Source: CAD feature listing. Evaluate the final solid. Frame: model axes, mm. A direction names the side the tool comes from. Give positions to 0.01 mm unless a question says otherwise; leave off trailing zeros. Loops run counter-clockwise (first coordinate to the right, second up) from the corner with the lowest first, then second, coordinate; pieces in that order, holes last. Notation, with made-up numbers: (-9.75, 9) -> (-2.75, 9) arc R26 cw to (-2.75, 44) -> close; hole circle Ø10 at (-26.75, 42.5). An arc over 180 degrees is marked (long way). Return JSON: item names as keys, results as strings. Group by question number.
(1) Cut plane A-A on x = -16.5. Return loops of the section in (y, z), then the cut area to 3 significant figures.
(2) Cut plane C-C on x = 0. Give the number of separate pieces and of enclosed holes in the cut face, then the cut area to 3 significant figures.
(3) Access query for faces 1 (the face through (52, 57, 10)), 2 (the face through (55, 10, 55)), 3 (the face through (-28, 57, 108)), 4 (the face through (23.944, 68.526, 104.028)). Directions: +Z, -Z, +X, -X, +Y, -Y. A direction counts if a zero-diameter tool reaches every point of the face in a straight line with its end or side. Return the directions, or none.
(4) Cut plane B-B on z = 52.5. Return loops of the section in (x, y), then the cut area to 3 significant figures.
(5) Cut plane D-D on y = -29.5. Return loops of the section in (x, z), then the cut area to 3 significant figures.
(6) Draft query along Y for faces 5 (the face through (-56.52, -9.85, 9.39)), 6 (the face through (-28, 57, 10)), 7 (the face through (-24.06, 67.65, 17)). Return one class per face: released by +Y, released by -Y, zero draft, split by the parting line, or undercut.
(7) Ray query, line 1 (X direction, y = 20.5, z = 59.5); line 2 (X direction, y = 65, z = 110); line 3 (Z direction, x = 20.5, y = 43.5). Return the intervals inside material, ascending. Write a range as from..to.
(8) Pin query (flat end, axial travel): pin 1 (6.5 mm diameter, centred on y = 58, z = 102, fed in from +X); pin 2 (7 mm diameter, centred on x = -4, y = -2, fed in from -Z); pin 3 (6 mm diameter, centred on y = 60.5, z = 110, fed in from -X). Return the tip coordinate at first contact, or that it passes through.
```python
from build123d import *

# Parameters (mm, degrees)
SKETCH_W        = 110
SKETCH_H        = 85
SKETCH_R        = 2.6
PAD_DEPTH       = 6
SKETCH001_R     = 12
POCKET_DEPTH    = 2
SKETCH002_W     = 110
SKETCH002_H     = 120
SKETCH002_W_2   = 75
SKETCH002_H_2   = 65
PAD001_DEPTH    = 6
PAD002_DEPTH    = 3
SKETCH004_W     = 8
SKETCH004_H     = 20
PAD003_DEPTH    = 22
SKETCH005_R     = 2.6
POCKET001_DEPTH = 110.001
FILLET_R        = 9.99
CHAMFER_SIZE    = 9.99
FILLET001_R     = 6
FILLET002_R     = 3
CHAMFER001_SIZE = 1.99
FILLET003_R     = 24


with BuildPart() as part:
    # Sketch → Pad (new body)
    with BuildSketch(Plane.XY):
        Rectangle(SKETCH_W, SKETCH_H)
        with Locations((0, -7.5)):
            Circle(SKETCH_R, mode=Mode.SUBTRACT)
    extrude(amount=PAD_DEPTH)

    # Sketch001 (on Face6 of Pad) → Pocket (cut)
    with BuildSketch(Plane(origin=(0, 0, 0), x_dir=(1, 0, 0), z_dir=(0, 0, -1))):
        with Locations((0, 7.5)):
            Circle(SKETCH001_R)
    extrude(amount=-POCKET_DEPTH, mode=Mode.SUBTRACT)

    # Sketch002 (on Face1 of Pocket) → Pad001 (join)
    with BuildSketch(Plane(origin=(0, 42.5, 0), x_dir=(-1, 0, 0), z_dir=(0, 1, 0))):
        with Locations((0, 60)):
            Rectangle(SKETCH002_W, SKETCH002_H)
        with Locations((0, 57.5)):
            Rectangle(SKETCH002_W_2, SKETCH002_H_2, mode=Mode.SUBTRACT)
    extrude(amount=PAD001_DEPTH)

    # Sketch003 (on Face15 of Pad001) → Pad002 (join)
    with BuildSketch(Plane.YZ.offset(55)):
        Polygon((-42.5, 6), (42.5, 120), (48.5, 120), (48.5, 0), (-42.5, 0), align=None)
        Polygon((42.5, 85), (-16.403509, 6), (42.5, 6), align=None, mode=Mode.SUBTRACT)
    pad002 = extrude(amount=PAD002_DEPTH)

    # Mirrored: Pad002 across YZ
    add(pad002.mirror(Plane.YZ))

    # Sketch004 (on Face13 of Mirrored) → Pad003 (join)
    with BuildSketch(Plane(origin=(0, 48.5, 0), x_dir=(-1, 0, 0), z_dir=(0, 1, 0))):
        with Locations((-24, 110)):
            Rectangle(SKETCH004_W, SKETCH004_H)
        with Locations((24, 110)):
            Rectangle(SKETCH004_W, SKETCH004_H)
        with Locations((-24, 10)):
            Rectangle(SKETCH004_W, SKETCH004_H)
        with Locations((24, 10)):
            Rectangle(SKETCH004_W, SKETCH004_H)
        with Locations((0, 10)):
            Rectangle(SKETCH004_W, SKETCH004_H)
        with Locations((0, 110)):
            Rectangle(SKETCH004_W, SKETCH004_H)
        with Locations((-48, 110)):
            Rectangle(SKETCH004_W, SKETCH004_H)
        with Locations((48, 110)):
            Rectangle(SKETCH004_W, SKETCH004_H)
        with Locations((-48, 10)):
            Rectangle(SKETCH004_W, SKETCH004_H)
        with Locations((48, 10)):
            Rectangle(SKETCH004_W, SKETCH004_H)
    extrude(amount=PAD003_DEPTH)

    # Sketch005 (on Face13 of Pad003) → Pocket001 (cut, through all)
    with BuildSketch(Plane.YZ.offset(52)):
        with Locations((60.5, 110)):
            Circle(SKETCH005_R)
        with Locations((60.5, 10)):
            Circle(SKETCH005_R)
    extrude(amount=-POCKET001_DEPTH, mode=Mode.SUBTRACT)

    # Fillet
    fillet_edges = [part.edges().sort_by_distance(p)[0] for p in [
        (48, 70.5, 0),
        (24, 70.5, 0),
        (0, 70.5, 0),
        (-24, 70.5, 0),
        (-48, 70.5, 0),
        (-48, 70.5, 20),
        (-24, 70.5, 20),
        (0, 70.5, 20),
        (24, 70.5, 20),
        (48, 70.5, 20),
        (48, 70.5, 100),
        (24, 70.5, 100),
        (0, 70.5, 100),
        (-24, 70.5, 100),
        (-48, 70.5, 100),
        (-48, 70.5, 120),
        (-24, 70.5, 120),
        (0, 70.5, 120),
        (24, 70.5, 120),
        (48, 70.5, 120),
    ]]
    fillet(fillet_edges, radius=FILLET_R)

    # Chamfer
    chamfer_edges = [part.edges().sort_by_distance(p)[0] for p in [
        (0, 48.5, 100),
        (-24, 48.5, 100),
        (-48, 48.5, 100),
        (24, 48.5, 100),
        (48, 48.5, 100),
    ]]
    chamfer(chamfer_edges, length=CHAMFER_SIZE)

    # Fillet001
    fillet001_edges = [part.edges().sort_by_distance(p)[0] for p in [
        (56.5, 42.5, 85),
        (56.5, -16.403509, 6),
        (0, 42.5, 6),
        (37.5, 45.5, 25),
        (-37.5, 45.5, 25),
        (-37.5, 45.5, 90),
        (37.5, 45.5, 90),
        (-56.5, 42.5, 85),
        (-56.5, -16.403509, 6),
    ]]
    fillet(fillet001_edges, radius=FILLET001_R)

    # Fillet002
    fillet002_edges = [part.edges().sort_by_distance(p)[0] for p in [
        (-58, -42.5, 3),
        (58, -42.5, 3),
        (-58, 45.5, 120),
        (58, 45.5, 120),
        (58, 48.5, 60),
        (-58, 48.5, 60),
        (58, 3, 0),
        (0, -42.5, 0),
        (-58, 3, 0),
    ]]
    fillet(fillet002_edges, radius=FILLET002_R)

    # Chamfer001
    chamfer001_edges = [part.edges().sort_by_distance(p)[0] for p in [
        (-12, -7.5, 0),
    ]]
    chamfer(chamfer001_edges, length=CHAMFER001_SIZE)

    # Fillet003
    fillet003_edges = [part.edges().sort_by_distance(p)[0] for p in [
        (48, 58.49, 100),
        (48, 60.51, 100),
        (24, 58.49, 100),
        (24, 60.51, 100),
        (0, 58.49, 100),
        (0, 60.51, 100),
        (-24, 58.49, 100),
        (-24, 60.51, 100),
        (-48, 58.49, 100),
        (-48, 60.51, 100),
    ]]
    fillet(fillet003_edges, radius=FILLET003_R)


solid = part.part
```
Answers:
{
 "1": {"outline": "(-42.5, 3) arc R3 ccw to (-39.5, 0) -> (48.5, 0) -> (48.5, 25) -> (42.5, 25) -> (42.5, 12) arc R6 cw to (36.5, 6) -> (-42.5, 6) -> close; (42.5, 90) -> (48.5, 90) -> (48.5, 120) -> (42.5, 120) -> close", "area": "846 mm²"},
 "2": {"separate pieces": "3", "enclosed holes": "2", "area": "1,580 mm²"},
 "3": {"face 1": "+Z, -Z, +X, +Y", "face 2": "+Z, -Y", "face 3": "+Z, -Z, +Y", "face 4": "+X, -X, +Y"},
 "4": {"outline": "(-58, -7.83) -> (-55, -7.83) -> (-55, 18.27) -> (-58, 18.27) -> close; (-58, 42.5) -> (-37.5, 42.5) -> (-37.5, 48.5) -> (-55, 48.5) arc R3 ccw to (-58, 45.5) -> close; (37.5, 42.5) -> (58, 42.5) -> (58, 45.5) arc R3 ccw to (55, 48.5) -> (37.5, 48.5) -> close; (55, -7.83) -> (58, -7.83) -> (58, 18.27) -> (55, 18.27) -> close", "area": "399 mm²"},
 "5": {"outline": "(-58, 3) arc R3 ccw to (-55, 0) -> (55, 0) arc R3 ccw to (58, 3) -> (58, 23.44) -> (55, 23.44) -> (55, 6) -> (-55, 6) -> (-55, 23.44) -> (-58, 23.44) -> close", "area": "797 mm²"},
 "6": {"face 5": "undercut", "face 6": "zero draft", "face 7": "released by +Y"},
 "7": {"line 1": "-58..-55, 55..58", "line 2": "-52..-44, -28..-20, -4..4, 20..28, 44..52", "line 3": "0..25, 90..120"},
 "8": {"pin 1": "x = 52", "pin 2": "z = 2", "pin 3": "x = -52"}
}
